Could you check a few things on this model? Use its own coordinates, in mm. Coordinates: 2 decimals unless noted, no trailing zeros. Write each loop counter-clockwise with the first axis right and the second up, starting at its lowest first coordinate (ties: lowest second). Pieces come first, ordered by that corner, then holes.
```python
from build123d import *

# Parameters (mm, degrees)
F1_DEPTH = 13.1
F3_R     = 2
F2_W     = 61
F2_H     = 1
F4_DEPTH = 2


# Not quite as in the source:
# - a feature names something its author has since deleted; it is built from what else it names


with BuildPart() as f1:
    # F0 (on Front) → F1 (new body)
    with BuildSketch(Plane.XZ):
        Polygon((22.7466161251, 39.9272560477), (-42.2533838749, 39.9272560477), (-42.2077284126, 38.4279510158), (22.7922715837, 38.4272560477), align=None)
    extrude(amount=F1_DEPTH)

    # F3
    f3_edges = [f1.edges().sort_by_distance(p)[0] for p in [
        (-42.230556, -13.1, 39.177604),
        (22.769444, -13.1, 39.177256),
        (22.769444, 0, 39.177256),
        (-42.230556, 0, 39.177604),
    ]]
    fillet(f3_edges, radius=F3_R)

    # F2 (on face) → F4 (join)
    with BuildSketch(Plane(origin=(0.0004108598, 0, 38.4274997341), x_dir=(0.9999999999, 0, -1.06918e-05), z_dir=(-1.06918e-05, 0, -0.9999999999))):
        with Locations((-9.7081392748, 12.6)):
            Rectangle(F2_W, F2_H)
    extrude(amount=F4_DEPTH)


solid = f1.part
```
1. Please list where these lines run through material, in increasing order: line 1 along Z through (x, y) = (-36, -11.75); line 2 along Y through (x, z) = (-12.5, 36.95); line 3 along X through (y, z) = (-3.5, 38.55).
Verdict:
line 1: z = 38.43 to 39.93
line 2: y = -13.1 to -12.1
line 3: x = -42.21 to 22.79
2. I want a section at A-A on y = -5.25. Please give me the cut outline in (x, z).
Verdict:
outline: (-42.25, 39.93) - (-42.21, 38.43) - (22.79, 38.43) - (22.75, 39.93) - close
3. For pin 1 (3 mm diameter, centred on x = 12.5, y = -10, fed in from -Z); pin 2 (1 mm diameter, centred on x = -2, z = 37.5, fed in from +Y); pin 3 (0.5 mm diameter, centred on y = -13, z = 37, fed in from -X), each with a flat end and sliding along its axis, tell me the tip position at first contact or that it passes through.
Verdict:
pin 1: stops at z = 38.43
pin 2: stops at y = -12.1
pin 3: stops at x = -40.21
4. I want a section at C-C on z = 37.85. Please give me the cut outline in (x, y), plus the area to 3 significant figures.
Verdict:
outline: (-40.21, -13.1) - (20.79, -13.1) - (20.79, -12.1) - (-40.21, -12.1) - close
area: 61.0 mm2
5. I want a section at B-B on x = 5.5. Please give me the cut outline in (y, z).
Verdict:
outline: (-13.1, 36.43) - (-12.1, 36.43) - (-12.1, 38.43) - (0, 38.43) - (0, 39.93) - (-13.1, 39.93) - close
